Work out the finished part from the listing and answer in its coordinate system (mm). A direction names the side the tool comes from. Coordinates: 2 decimals unless noted, no trailing zeros. Order: outer loops, then holes, each group sorted by start corner. A loop starts at its lowest first (then second) coordinate and runs counter-clockwise, first axis right, second up. Notation, with made-up numbers: M 14.25,18.25 L 20.25,18.25 A18 ccw 20.25,33.25 Z; hole C -2.75,41 d1. An arc over 180 degrees is marked long. Write item = value, one per line. Start each with the question number.
Q1. Find section A-A on y = 82. Give the vertices of the cut face in (x, z).
Q2. Straight lines are drawn through the part: line 1 along X through (y, z) = (6.5, 2.2); line 2 along Y through (x, z) = (37, 1.8); line 3 along X through (y, z) = (73, 3.6). For each, find the intervals that lie inside material, in ascending order.
Q3. Find section B-B on z = 4.25. Give the number of separate pieces and of enclosed holes in the cut face, and give its area (3 significant figures).
Q4. Each of these flat-tipped pins is pushed along its axis until it touches: P1, Ø1, axis at y = 6, z = 3.5, coming from the +X side; P2, Ø0.7, axis at x = 87.5, z = 4, coming from the +Y side; P3, Ø1, axis at x = 0.5, z = 3.5, coming from the -Y side. Where does it stop, or does it pass through?
Q5. Find section D-D on x = 57. Give the vertices of the cut face in (y, z), and give its area (3 significant figures).
Q6. Determine the mould class of faces 5 (the flat face through (83.065, -1, 3)), 6 (the flat face through (119.298, 47.406, 3.153)), 7 (the flat face through (-13, 10.979, 3)) for opening direction Y: released by +Y, released by -Y, zero draft, split by the parting line, or undercut.
Q7. A tool of negligible diameter and unlimited length cuts with its end or side. For faces 1 (the flat face through (96, -4.896, 3)), 2 (the flat face through (1, -4.896, 3)), 3 (the flat face through (-7.232, 5, 3)), 4 (the flat face through (80.964, 77.658, 3.153)), from which of +Z, -Z, +X, -X, +Y, -Y can it reach the whole face along a straight path? Write none if from no direction.
Q8. Find section C-C on x = 26. Give the vertices of the cut face in (y, z).
```python
from build123d import *

# Parameters (mm, degrees)
BOSS_EXTRUDE2_DEPTH = 6.35
SCALE1_DEPTH        = 6.35
SCALE1_2_DEPTH      = 1.587500269
SCALE1_START        = 4.762500269
SCALE1_3_DEPTH      = 1.587499731
SCALE1_START_2      = 1.587500269
SCALE1_4_DEPTH      = 3.175
SKETCH2_W           = 3.175
SKETCH2_H           = 3.175
CUT_EXTRUDE2_DEPTH  = 3.175
SKETCH3_W           = 20.32
SKETCH3_H           = 3.175
BOSS_EXTRUDE3_DEPTH = 3.175
CUT_EXTRUDE3_DEPTH  = 3.175


# Read off the part's stored shape, not the designer's step: Scale1
with BuildPart() as part:
    # Sketch1 → Boss-Extrude2 (new body)
    with BuildSketch(Plane.XY):
        with BuildLine():
            Line((83.827808052, -44.105116896), (-89.955824252, -44.105116896))
            add(Edge.make_bspline(
                [(-89.955824252, -44.105116896), (-138.279146298, 17.577773588), (-90.448185334, 121.033367978), (0, 109.592549188)],
                knots=[0, 0, 0, 0, 1, 1, 1, 1], degree=3))
            Line((0, 109.592549188), (44.001127073, 142.976601592))
            Line((44.001127073, 142.976601592), (83.827808052, 99.113432677))
            Line((83.827808052, 99.113432677), (151.46035168, 143.51342315))
            Line((151.46035168, 143.51342315), (168.705700605, 55.742873106))
            Line((168.705700605, 55.742873106), (219.688100022, 65.389167163))
            Line((219.688100022, 65.389167163), (164.044175748, -44.105116896))
            Line((164.044175748, -44.105116896), (83.827808052, -44.105116896))
        make_face()
        with BuildLine():
            Line((108.479325939, 0.038399309), (131.217832103, 46.925099923))
            Line((131.217832103, 46.925099923), (105.101551368, 40.233461811))
            add(Edge.make_bspline(
                [(108.479325939, 0.038399309), (109.348375822, 7.243418902), (109.431703621, 20.845994783), (106.837891987, 34.226883905), (105.101551368, 40.233461811)],
                knots=[0.221169561, 0.221169561, 0.221169561, 0.221169561, 0.320684156, 0.405876818, 0.405876818, 0.405876818, 0.405876818], degree=3))
        make_face(mode=Mode.SUBTRACT)
        with BuildLine():
            Line((31.501577026, 104.663344036), (45.60523641, 113.478131151))
            Line((45.60523641, 113.478131151), (58.141193688, 93.420599506))
            add(Edge.make_bspline(
                [(58.141193688, 93.420599506), (46.052907541, 102.061530026), (31.501577026, 104.663344036)],
                knots=[0, 0, 0, 1, 1, 1], degree=2))
        make_face(mode=Mode.SUBTRACT)
    extrude(amount=BOSS_EXTRUDE2_DEPTH)

    # Scale1 outline → Scale1 (cut)
    # profile 1 of 3: a face of its own
    with BuildSketch(Plane.XY):
        with BuildLine():
            Line((44.001127073, 142.976601592), (0, 109.592549188))
            add(Edge.make_bspline(
                [(0, 109.592549188), (-90.448185334, 121.033367978), (-138.279146298, 17.577773588), (-89.955824252, -44.105116896)],
                knots=[0, 0, 0, 0, 1, 1, 1, 1], degree=3))
            Line((-89.955824252, -44.105116896), (164.044175748, -44.105116896))
            Line((164.044175748, -44.105116896), (219.688100022, 65.389167163))
            Line((219.688100022, 65.389167163), (168.705700605, 55.742873106))
            Line((168.705700605, 55.742873106), (151.46035168, 143.51342315))
            Line((151.46035168, 143.51342315), (83.827808052, 99.113432677))
            Line((83.827808052, 99.113432677), (44.001127073, 142.976601592))
        make_face()
        with BuildLine():
            add(Edge.make_bspline(
                [(22.378427384, 71.952774895), (-22.845665283, 77.67318429), (-46.761145765, 25.945387095), (-22.599484742, -4.896058147)],
                knots=[0, 0, 0, 0, 1, 1, 1, 1], degree=3))
            Line((22.378427384, 71.952774895), (44.378990921, 88.644801097))
            Line((44.378990921, 88.644801097), (64.29233141, 66.713216639))
            Line((64.29233141, 66.713216639), (98.108603224, 88.913211876))
            Line((98.108603224, 88.913211876), (106.731277687, 45.027936854))
            Line((106.731277687, 45.027936854), (132.222477396, 49.851083882))
            Line((132.222477396, 49.851083882), (130.663317047, 46.783019429))
            Line((130.663317047, 46.783019429), (131.217832103, 46.925099923))
            Line((131.217832103, 46.925099923), (108.479325939, 0.038399309))
            add(Edge.make_bspline(
                [(108.864671926, 3.888362517), (108.762049288, 2.601843236), (108.633688525, 1.318171025), (108.479325939, 0.038399309)],
                knots=[0.388200813, 0.388200813, 0.388200813, 0.388200813, 0.405876818, 0.405876818, 0.405876818, 0.405876818], degree=3))
            Line((108.864671926, 3.888362517), (104.400515258, -4.896058147))
            Line((104.400515258, -4.896058147), (-22.599484742, -4.896058147))
        make_face(mode=Mode.SUBTRACT)
        with BuildLine():
            add(Edge.make_bspline(
                [(31.501577026, 104.663344036), (46.052907541, 102.061530026), (58.141193688, 93.420599506)],
                knots=[0, 0, 0, 1, 1, 1], degree=2))
            Line((31.501577026, 104.663344036), (45.60523641, 113.478131151))
            Line((45.60523641, 113.478131151), (58.141193688, 93.420599506))
        make_face(mode=Mode.SUBTRACT)
    # profile 2 of 3: a face of its own
    with BuildSketch(Plane.XY):
        with BuildLine():
            Line((45.18104559, 73.895565876), (38.129215897, 69.488172319))
            add(Edge.make_bspline(
                [(38.129215897, 69.488172319), (45.404881155, 68.187265314), (51.449024229, 63.866800054)],
                knots=[0, 0, 0, 1, 1, 1], degree=2))
            Line((51.449024229, 63.866800054), (45.18104559, 73.895565876))
        make_face()
    # profile 3 of 3: a face of its own
    with BuildSketch(Plane.XY):
        with BuildLine():
            Line((87.987343436, 40.619050262), (74.929203069, 37.273231206))
            add(Edge.make_bspline(
                [(74.929203069, 37.273231206), (75.797373378, 34.269942253), (77.094279195, 27.579497692), (77.052615295, 20.778209752), (76.618090354, 17.175699955)],
                knots=[0.221169561, 0.221169561, 0.221169561, 0.221169561, 0.306362223, 0.405876818, 0.405876818, 0.405876818, 0.405876818], degree=3))
            Line((76.618090354, 17.175699955), (87.987343436, 40.619050262))
        make_face()
    extrude(amount=SCALE1_DEPTH, mode=Mode.SUBTRACT)

    # Scale1 2 outline → Scale1 2 (cut)
    with BuildSketch(Plane.XY):
        with BuildLine():
            Line((44.378990921, 88.644801097), (22.378427384, 71.952774895))
            add(Edge.make_bspline(
                [(22.378427384, 71.952774895), (-22.845665283, 77.67318429), (-46.761145765, 25.945387095), (-22.599484742, -4.896058147)],
                knots=[0, 0, 0, 0, 1, 1, 1, 1], degree=3))
            Line((-22.599484742, -4.896058147), (104.400515258, -4.896058147))
            Line((104.400515258, -4.896058147), (108.864671926, 3.888362517))
            add(Edge.make_bspline(
                [(105.101551368, 40.233461811), (106.837891987, 34.226883905), (109.183482579, 22.126511148), (109.339807105, 9.844851123), (108.864671926, 3.888362517)],
                knots=[0.221169561, 0.221169561, 0.221169561, 0.221169561, 0.306362223, 0.388200813, 0.388200813, 0.388200813, 0.388200813], degree=3))
            Line((105.101551368, 40.233461811), (130.663317047, 46.783019429))
            Line((130.663317047, 46.783019429), (132.222477396, 49.851083882))
            Line((132.222477396, 49.851083882), (106.731277687, 45.027936854))
            Line((106.731277687, 45.027936854), (98.108603224, 88.913211876))
            Line((98.108603224, 88.913211876), (64.29233141, 66.713216639))
            Line((64.29233141, 66.713216639), (44.378990921, 88.644801097))
        make_face()
        with BuildLine():
            add(Edge.make_bspline(
                [(74.929203069, 37.273231206), (75.797373378, 34.269942253), (77.094279195, 27.579497692), (77.052615295, 20.778209752), (76.618090354, 17.175699955)],
                knots=[0.221169561, 0.221169561, 0.221169561, 0.221169561, 0.306362223, 0.405876818, 0.405876818, 0.405876818, 0.405876818], degree=3))
            Line((74.929203069, 37.273231206), (87.987343436, 40.619050262))
            Line((87.987343436, 40.619050262), (76.618090354, 17.175699955))
        make_face(mode=Mode.SUBTRACT)
        with BuildLine():
            add(Edge.make_bspline(
                [(38.129215897, 69.488172319), (45.404881155, 68.187265314), (51.449024229, 63.866800054)],
                knots=[0, 0, 0, 1, 1, 1], degree=2))
            Line((38.129215897, 69.488172319), (45.18104559, 73.895565876))
            Line((45.18104559, 73.895565876), (51.449024229, 63.866800054))
        make_face(mode=Mode.SUBTRACT)
    extrude(amount=SCALE1_2_DEPTH, mode=Mode.SUBTRACT)

    # Scale1 3 outline → Scale1 3 (cut)
    with BuildSketch(Plane.XY.offset(SCALE1_START)):
        with BuildLine():
            Line((44.378990921, 88.644801097), (22.378427384, 71.952774895))
            add(Edge.make_bspline(
                [(22.378427384, 71.952774895), (-22.845665283, 77.67318429), (-46.761145765, 25.945387095), (-22.599484742, -4.896058147)],
                knots=[0, 0, 0, 0, 1, 1, 1, 1], degree=3))
            Line((-22.599484742, -4.896058147), (104.400515258, -4.896058147))
            Line((104.400515258, -4.896058147), (108.864671926, 3.888362517))
            add(Edge.make_bspline(
                [(105.101551368, 40.233461811), (106.837891987, 34.226883905), (109.183482579, 22.126511148), (109.339807105, 9.844851123), (108.864671926, 3.888362517)],
                knots=[0.221169561, 0.221169561, 0.221169561, 0.221169561, 0.306362223, 0.388200813, 0.388200813, 0.388200813, 0.388200813], degree=3))
            Line((105.101551368, 40.233461811), (130.663317047, 46.783019429))
            Line((130.663317047, 46.783019429), (132.222477396, 49.851083882))
            Line((132.222477396, 49.851083882), (106.731277687, 45.027936854))
            Line((106.731277687, 45.027936854), (98.108603224, 88.913211876))
            Line((98.108603224, 88.913211876), (64.29233141, 66.713216639))
            Line((64.29233141, 66.713216639), (44.378990921, 88.644801097))
        make_face()
        with BuildLine():
            add(Edge.make_bspline(
                [(74.929203069, 37.273231206), (75.797373378, 34.269942253), (77.094279195, 27.579497692), (77.052615295, 20.778209752), (76.618090354, 17.175699955)],
                knots=[0.221169561, 0.221169561, 0.221169561, 0.221169561, 0.306362223, 0.405876818, 0.405876818, 0.405876818, 0.405876818], degree=3))
            Line((74.929203069, 37.273231206), (87.987343436, 40.619050262))
            Line((87.987343436, 40.619050262), (76.618090354, 17.175699955))
        make_face(mode=Mode.SUBTRACT)
        with BuildLine():
            add(Edge.make_bspline(
                [(38.129215897, 69.488172319), (45.404881155, 68.187265314), (51.449024229, 63.866800054)],
                knots=[0, 0, 0, 1, 1, 1], degree=2))
            Line((38.129215897, 69.488172319), (45.18104559, 73.895565876))
            Line((45.18104559, 73.895565876), (51.449024229, 63.866800054))
        make_face(mode=Mode.SUBTRACT)
    extrude(amount=SCALE1_3_DEPTH, mode=Mode.SUBTRACT)

    # Scale1 4 outline → Scale1 4 (add)
    with BuildSketch(Plane.XY.offset(SCALE1_START_2)):
        with BuildLine():
            add(Edge.make_bspline(
                [(105.101551368, 40.233461811), (106.837891987, 34.226883905), (109.183482579, 22.126511148), (109.339807105, 9.844851123), (108.864671926, 3.888362517)],
                knots=[0.221169561, 0.221169561, 0.221169561, 0.221169561, 0.306362223, 0.388200813, 0.388200813, 0.388200813, 0.388200813], degree=3))
            Line((108.864671926, 3.888362517), (130.663317047, 46.783019429))
            Line((130.663317047, 46.783019429), (105.101551368, 40.233461811))
        make_face()
    extrude(amount=SCALE1_4_DEPTH)

    # Sketch2 → Cut-Extrude2 (cut)
    with BuildSketch(Plane.XY.offset(4.762500269)):
        with Locations((-13.391984742, 9.391441853)):
            Rectangle(SKETCH2_W, SKETCH2_H)
        with Locations((95.193015258, 9.391441853)):
            Rectangle(SKETCH2_W, SKETCH2_H)
    extrude(amount=-CUT_EXTRUDE2_DEPTH, mode=Mode.SUBTRACT)

    # Sketch3 → Boss-Extrude3 (add)
    with BuildSketch(Plane.XZ.offset(4.896058147)):
        with Locations((12.960515258, 3.175000269)):
            Rectangle(SKETCH3_W, SKETCH3_H)
        with Locations((68.840515258, 3.175000269)):
            Rectangle(SKETCH3_W, SKETCH3_H)
    extrude(amount=BOSS_EXTRUDE3_DEPTH)

    # Sketch4 → Cut-Extrude3 (cut)
    with BuildSketch(Plane.XY.offset(4.762500269)):
        Polygon((-7.232484742, 7.803941853), (1.149515258, 7.803941853), (1.149515258, 2.723941853), (-1.263484742, 2.723941853), (-1.263484742, -4.896058147), (-4.819484742, -4.896058147), (-4.819484742, 2.723941853), (-7.232484742, 2.723941853), align=None)
        Polygon((36.709515258, 7.803941853), (45.091515258, 7.803941853), (45.091515258, 2.723941853), (42.678515258, 2.723941853), (42.678515258, -4.896058147), (39.122515258, -4.896058147), (39.122515258, 2.723941853), (36.709515258, 2.723941853), align=None)
        Polygon((80.651515258, 7.803941853), (89.033515258, 7.803941853), (89.033515258, 2.723941853), (86.620515258, 2.723941853), (86.620515258, -4.896058147), (83.064515258, -4.896058147), (83.064515258, 2.723941853), (80.651515258, 2.723941853), align=None)
    extrude(amount=-CUT_EXTRUDE3_DEPTH, mode=Mode.SUBTRACT)


solid = part.part
```
Findings below:
q1.outline = M 35.62,1.59 L 50.41,1.59 L 50.41,4.76 L 35.62,4.76 Z; M 87.58,1.59 L 99.47,1.59 L 99.47,4.76 L 87.58,4.76 Z
q2.line_1 = -29.09 to -7.23, 1.15 to 36.71, 45.09 to 80.65, 89.03 to 110.19
q2.line_2 = -4.9 to 2.72, 7.8 to 83.05
q2.line_3 = 23.76 to 43.75, 45.74 to 58.58, 73.87 to 101.24
q3.separate_pieces = 1
q3.enclosed_holes = 4
q3.area = 10,900 mm^2
q4.P1 = 110.19
q4.P2 = 82.18
q4.P3 = -4.9
q5.outline = M -4.9,1.59 L 74.74,1.59 L 74.74,4.76 L -4.9,4.76 Z
q5.area = 253 mm^2
q6.face_5 = zero draft
q6.face_6 = released by +Y
q6.face_7 = undercut
q7.face_1 = +Z, -Z, +X, -Y
q7.face_2 = +Z, -Z, -X, -Y
q7.face_3 = +Z, -Z
q7.face_4 = +Z, -Z, +Y
q8.outline = M -4.9,1.59 L 74.7,1.59 L 74.7,4.76 L -4.9,4.76 Z
